Source: CAD feature listing. Evaluate the final solid. Frame: model axes, mm. A direction names the side the tool comes from. Give positions to 0.01 mm unless a question says otherwise; leave off trailing zeros. Order: outer loops, then holes, each group sorted by start corner. A loop starts at its lowest first (then second) coordinate and runs counter-clockwise, first axis right, second up. Notation, with made-up numbers: (-32, -20.5) - (-9, -20.5) arc R31 cw to (-9, 4.5) - close; hole circle Ø1 at (-1.75, -7). An arc over 180 degrees is marked (long way). One line per item, written item: value. Start each with the question number.
from build123d import *

# Parameters (mm, degrees)
SKETCH2_W                    = 203.2
SKETCH2_H                    = 88.9
BASE_FLANGE1_DEPTH           = 6.35
EDGE_FLANGE1_START           = -101.6
EDGE_FLANGE1_DEPTH           = 203.2
EDGE_FLANGE1_2_DEPTH         = 203.2
EDGE_FLANGE2_STRIP_W         = 31.75
EDGE_FLANGE2_STRIP_H         = 6.35
EDGE_FLANGE2_STRIP_CUT_DEPTH = 203.2
EDGE_FLANGE2_DEPTH           = 203.2
SKETCH13_R                   = 33.3375
SKETCH13_R_2                 = 3
CUT_EXTRUDE1_DEPTH           = 322.27645633
EDGE_FLANGE3_START           = -101.6
EDGE_FLANGE3_DEPTH           = 203.2
EDGE_FLANGE3_2_DEPTH         = 203.2
SKETCH17_R                   = 6.35
CUT_EXTRUDE2_DEPTH           = 373.253425916
SKETCH18_R                   = 4.7625
CUT_EXTRUDE3_DEPTH           = 370.310259163
BREAK_CORNER1_START          = -323.104570995
BREAK_CORNER1_OUTLINE_W      = 145.614442934
BREAK_CORNER1_OUTLINE_H      = 10
BREAK_CORNER1_DEPTH          = 4.490128061
BREAK_CORNER1_START_2        = -183.910601118
BREAK_CORNER1_2_OUTLINE_W    = 5.385557066
BREAK_CORNER1_2_OUTLINE_H    = 10
BREAK_CORNER1_2_DEPTH        = 8.980256121
SKETCH19_R                   = 6.35
CUT_EXTRUDE4_DEPTH           = 391.404403674
SKETCH20_R                   = 4.7625
CUT_EXTRUDE5_DEPTH           = 367.686034552


# Read off the part's stored shape, not the designer's step: Edge-Flange1, Edge-Flange3, Break-Corner1
# Sheet-metal steps are written as plain solids
with BuildPart() as part:
    # Sketch2 → Base-Flange1 (new body)
    with BuildSketch(Plane.XY):
        Rectangle(SKETCH2_W, SKETCH2_H)
    extrude(amount=-BASE_FLANGE1_DEPTH)

    # Edge-Flange1 outline → Edge-Flange1 (cut)
    with BuildSketch(Plane.YZ.offset(EDGE_FLANGE1_START)):
        with BuildLine():
            Line((44.45, 0), (44.419989189, 0))
            ThreePointArc((44.419989189, 0), (40.938994382, -4.602129933), (35.439733068, -6.35))
            Line((35.439733068, -6.35), (44.45, -6.35))
            Line((44.45, -6.35), (44.45, 0))
        make_face()
    extrude(amount=EDGE_FLANGE1_DEPTH, mode=Mode.SUBTRACT)

    # Edge-Flange1 2 outline → Edge-Flange1 2 (add)
    with BuildSketch(Plane.YZ.offset(EDGE_FLANGE1_START)):
        with BuildLine():
            ThreePointArc((44.419989189, 0), (44.537007132, 0.352726165), (44.640176563, 0.709748595))
            Line((44.640176563, 0.709748595), (107.504969662, 235.324350447))
            Line((107.504969662, 235.324350447), (101.371340665, 236.967851383))
            Line((101.371340665, 236.967851383), (38.506547566, 2.353249532))
            ThreePointArc((38.506547566, 2.353249532), (37.372550605, 0.656103145), (35.439733068, 0))
            Line((35.439733068, 0), (44.419989189, 0))
        make_face()
    extrude(amount=EDGE_FLANGE1_2_DEPTH)

    # Edge-Flange2 strip (across the edge) → Edge-Flange2 strip cut (cut)
    with BuildSketch(Plane(origin=(-101.6, 107.504969662, 235.324350447), x_dir=(0, -0.25881904510252135, -0.9659258262890682), z_dir=(1, 0, 0))):
        with Locations((-6.35, -3.175)):
            Rectangle(EDGE_FLANGE2_STRIP_W, EDGE_FLANGE2_STRIP_H)
    extrude(amount=EDGE_FLANGE2_STRIP_CUT_DEPTH, mode=Mode.SUBTRACT)

    # Edge-Flange2 section (across the edge) → Edge-Flange2 (add)
    with BuildSketch(Plane(origin=(-101.6, 107.504969662, 235.324350447), x_dir=(0, -0.25881904510252135, -0.9659258262890682), z_dir=(1, 0, 0))):
        with BuildLine():
            Line((0, 3.175), (0, 133.35))
            Line((0, 133.35), (6.35, 133.35))
            Line((6.35, 133.35), (6.35, 3.175))
            ThreePointArc((6.35, 3.175), (7.27993597, 0.92993597), (9.525, 0))
            Line((9.525, 0), (9.525, -6.35))
            ThreePointArc((9.525, -6.35), (2.789807909, -3.560192091), (0, 3.175))
        make_face()
    extrude(amount=EDGE_FLANGE2_DEPTH)

    # Sketch13 → Cut-Extrude1 (cut, through all)
    with BuildSketch(Plane(origin=(0, 66.032555063, 246.436850447), x_dir=(1, 0, 0), z_dir=(0, 0.25881904510252135, 0.9659258262890682))):
        with Locations(Location((0, 107.070402979, 0), (0, 0, 270))):
            Circle(SKETCH13_R)
        with Locations(Location((35.074028853, 86.820402979, 0), (0, 0, 270))):
            Circle(SKETCH13_R_2)
        with Locations(Location((0, 66.570402979, 0), (0, 0, 270))):
            Circle(SKETCH13_R_2)
        with Locations(Location((-35.074028853, 86.820402979, 0), (0, 0, 270))):
            Circle(SKETCH13_R_2)
        with Locations(Location((-35.074028853, 127.320402979, 0), (0, 0, 270))):
            Circle(SKETCH13_R_2)
        with Locations(Location((35.074028853, 127.320402979, 0), (0, 0, 270))):
            Circle(SKETCH13_R_2)
        with Locations(Location((0, 147.570402979, 0), (0, 0, 270))):
            Circle(SKETCH13_R_2)
    extrude(amount=-CUT_EXTRUDE1_DEPTH, mode=Mode.SUBTRACT)

    # Edge-Flange3 outline → Edge-Flange3 (cut)
    with BuildSketch(Plane.YZ.offset(EDGE_FLANGE3_START)):
        with BuildLine():
            Line((236.311178597, 200.810830783), (236.28219038, 200.818598152))
            ThreePointArc((236.28219038, 200.818598152), (231.72868872, 197.274229745), (225.964428129, 197.009230469))
            Line((225.964428129, 197.009230469), (234.667677661, 194.677201786))
            Line((234.667677661, 194.677201786), (236.311178597, 200.810830783))
        make_face()
    extrude(amount=EDGE_FLANGE3_DEPTH, mode=Mode.SUBTRACT)

    # Edge-Flange3 2 outline → Edge-Flange3 2 (add)
    with BuildSketch(Plane.YZ.offset(EDGE_FLANGE3_START)):
        with BuildLine():
            ThreePointArc((236.28219038, 200.818598152), (236.486513283, 201.129018993), (236.678571505, 201.447173965))
            Line((236.678571505, 201.447173965), (267.949176724, 255.609450989))
            Line((267.949176724, 255.609450989), (262.44991541, 258.784450989))
            Line((262.44991541, 258.784450989), (231.179310191, 204.622173965))
            ThreePointArc((231.179310191, 204.622173965), (229.644699431, 203.276356449), (227.607929065, 203.142859466))
            Line((227.607929065, 203.142859466), (236.28219038, 200.818598152))
        make_face()
    extrude(amount=EDGE_FLANGE3_2_DEPTH)

    # Sketch17 → Cut-Extrude2 (cut, through all)
    with BuildSketch(Plane(origin=(0, 84.780482228, -48.948034236), x_dir=(1, 0, 0), z_dir=(0, -0.8660254037844363, 0.5000000000000042))):
        with Locations(Location((-69.85, 336.288866366, 0), (0, 0, 270))):
            Circle(SKETCH17_R)
        with Locations(Location((69.85, 336.288866366, 0), (0, 0, 270))):
            Circle(SKETCH17_R)
    extrude(amount=-CUT_EXTRUDE2_DEPTH, mode=Mode.SUBTRACT)

    # Sketch18 → Cut-Extrude3 (cut, through all)
    with BuildSketch(Plane(origin=(0, 35.338785602, -9.468999064), x_dir=(1, 0, 0), z_dir=(0, -0.9659258262890673, 0.2588190451025248))):
        with Locations(Location((-44.45, 196.339070344, 0), (0, 0, 270))):
            Circle(SKETCH18_R)
        with Locations(Location((44.45, 196.339070344, 0), (0, 0, 270))):
            Circle(SKETCH18_R)
    extrude(amount=-CUT_EXTRUDE3_DEPTH, mode=Mode.SUBTRACT)

    # Break-Corner1 outline → Break-Corner1 (cut)
    with BuildSketch(Plane(origin=(0, 0, 0), x_dir=(0.7071067811865475, 0.35355339059327684, 0.6123724356957928), z_dir=(0.7071067811865476, -0.3535533905932768, -0.6123724356957927)).offset(BREAK_CORNER1_START)):
        with Locations((245.807221467, -101)):
            Rectangle(BREAK_CORNER1_OUTLINE_W, BREAK_CORNER1_OUTLINE_H)
    extrude(amount=BREAK_CORNER1_DEPTH, mode=Mode.SUBTRACT)

    # Break-Corner1 2 outline → Break-Corner1 2 (cut)
    with BuildSketch(Plane(origin=(0, 0, 0), x_dir=(0.7071067811865475, 0.35355339059327684, 0.6123724356957928), z_dir=(0.7071067811865476, -0.3535533905932768, -0.6123724356957927)).offset(BREAK_CORNER1_START_2)):
        with Locations((321.307221467, -101)):
            Rectangle(BREAK_CORNER1_2_OUTLINE_W, BREAK_CORNER1_2_OUTLINE_H)
    extrude(amount=BREAK_CORNER1_2_DEPTH, mode=Mode.SUBTRACT)

    # Sketch19 → Cut-Extrude4 (cut, through all)
    with BuildSketch(Plane(origin=(0, 0, -6.35), x_dir=(-1, 0, 0), z_dir=(0, 0, -1))):
        with Locations((-88.9, 19.05)):
            Circle(SKETCH19_R)
        with Locations((-88.9, -19.05)):
            Circle(SKETCH19_R)
        with Locations((88.9, -19.05)):
            Circle(SKETCH19_R)
        with Locations((88.9, 19.05)):
            Circle(SKETCH19_R)
    extrude(amount=-CUT_EXTRUDE4_DEPTH, mode=Mode.SUBTRACT)

    # Sketch20 → Cut-Extrude5 (cut, through all)
    with BuildSketch(Plane(origin=(0, 41.472414599, -11.1125), x_dir=(1, 0, 0), z_dir=(0, 0.9659258262890673, -0.2588190451025248))):
        with Locations(Location((63.364615818, -153.530201243, 0), (0, 0, 270))):
            Circle(SKETCH20_R)
        with Locations(Location((63.364615818, -90.030201243, 0), (0, 0, 270))):
            Circle(SKETCH20_R)
        with Locations(Location((-63.364615818, -90.030201243, 0), (0, 0, 270))):
            Circle(SKETCH20_R)
        with Locations(Location((-63.364615818, -153.530201243, 0), (0, 0, 270))):
            Circle(SKETCH20_R)
    extrude(amount=-CUT_EXTRUDE5_DEPTH, mode=Mode.SUBTRACT)


solid = part.part
1. Section B-B on x = -88.9. Return the cut outline in (y, z) (3 decimals), then the cut area to 3 significant figures.
2. Draft query along X for faces 4 (the flat face through (-98.47, 263.55, 254.43)), 5 (the cylindrical face through (82.843, 20.957, -3.219)), 6 (the flat face through (-24, 142.3, 226)), 7 (the flat face through (98.381, 263.673, 254.464)). Return one class per face: pulls with the +X half, pulls with the -X half, needs draft (parallel to the pull), parting line crosses it, or undercut.
3. Section A-A on y = -19.05. Return the cut outline in (x, z).
4. Section C-C on z = 122.5. Return the cut outline in (x, y), then the cut area to 3 significant figures.
5. Set-up query: faces 1 (the flat face through (-1, -4, 0)), 2 (the flat face through (-1.42, 247.03, 232.08)), 3 (the cylindrical face through (-38.003, 188.833, 210.292)). Return all of +Z, -Z, +X, -X, +Y, -Y with unobstructed straight access to the full face (end or side cutting, diameter ignored); none if empty.
6. Ray query, L1, parallel to Y at x = -88, z = -2; L2, parallel to X at y = 19, z = -2; L3, parallel to Y at x = -88.9, z = -1.5. Return the intervals inside material, ascending.
7. Contact query for flat-ended pins moving along their axis: pin 1 Ø2 at (x, z) = (77.5, 47) entering from +Y; pin 2 Ø14.5 at (x, y) = (-88.9, -19.05) entering from -Z; pin 3 Ø2 at (x, y) = (0, 207) entering from -Z; pin 4 Ø24 at (x, y) = (-14.5, 13.5) entering from +Z. Output: stop coordinate, or through.
Data:
1. outline: (-44.45, -6.35) - (-25.4, -6.35) - (-25.4, 0) - (-44.45, 0) - close; (-12.7, -6.35) - (12.7, -6.35) - (12.7, 0) - (-12.7, 0) - close; (25.4, -6.35) - (35.44, -6.35) arc R9.525 ccw to (44.64, 0.71) - (105.04, 226.124) arc R3.175 cw to (108.928, 228.369) - (225.964, 197.009) arc R9.525 ccw to (236.679, 201.447) - (267.949, 255.609) - (262.45, 258.784) - (231.179, 204.622) arc R3.175 cw to (227.608, 203.143) - (110.572, 234.503) arc R9.525 ccw to (98.906, 227.767) - (38.507, 2.353) arc R3.175 cw to (35.44, 0) - (25.4, 0) - close
1. area: 3,160 mm2
2. face 4: pulls with the -X half
2. face 5: undercut
2. face 6: needs draft
2. face 7: pulls with the +X half
3. outline: (-101.6, -6.35) - (-95.25, -6.35) - (-95.25, 0) - (-101.6, 0) - close; (-82.55, -6.35) - (82.55, -6.35) - (82.55, 0) - (-82.55, 0) - close; (95.25, -6.35) - (101.6, -6.35) - (101.6, 0) - (95.25, 0) - close
4. outline: (-101.6, 70.7) - (101.6, 70.7) - (101.6, 77.27) - (-101.6, 77.27) - close
4. area: 1,340 mm2
5. face 1: +Z, +X, -X, -Y
5. face 2: +Z, +X, -X
5. face 3: none
6. L1: y = -44.45 to -25.34, -12.76 to 12.76, 25.34 to 43.44
6. L2: x = -101.6 to -95.25, -82.55 to 82.55, 95.25 to 101.6
6. L3: y = -44.45 to -25.4, -12.7 to 12.7, 25.4 to 43.74
7. pin 1: stops at y = 57.31
7. pin 2: stops at z = -6.35
7. pin 3: passes through
7. pin 4: stops at z = 0
